Answer from the drawing. Dimensions are ordinates in mm from the lowest x, y and z of the part. Round coordinates to 2 decimals unless told otherwise and drop trailing zeros. Write each loop counter-clockwise with the first axis right and the second up, starting at its lowest first coordinate (ties: lowest second). Pieces come first, ordered by that corner, then holes. Notation, with made-up numbers: (10.25, 27.5) -> (48.25, 27.5) arc R9 ccw to (48.25, 38.5) -> close; hole circle Ø3 at (88.5, -13.5). An arc over 180 degrees is marked (long way). Return JSON: item names as keys, results as strings. Group by question number.
(1) A cutting plane is placed at C-C on z = 10.25. Give the vertices of the cut face in (x, y), then the cut area to 3 significant figures.
(2) Given pin 1 (6 mm diameter, centred on y = 1.5, z = 7, fed in from +X); pin 2 (1.5 mm diameter, centred on x = 4.5, z = 16.5, fed in from -Y); pin 3 (3 mm diameter, centred on x = 3, y = 13.5, fed in from +Z) (1 decimal), each flat-ended and moving along its own axis, determine where each tip first touches the part or whether it passes through.
(3) A cutting plane is placed at D-D on z = 21.75. Give the vertices of the cut face in (x, y).
(4) Straight lines are drawn through the part: line 1 (X direction, y = 7.62, z = 1.2); line 2 (Y direction, x = 14, z = 15) (1 decimal). For each, find the intervals that lie inside material, in ascending order.
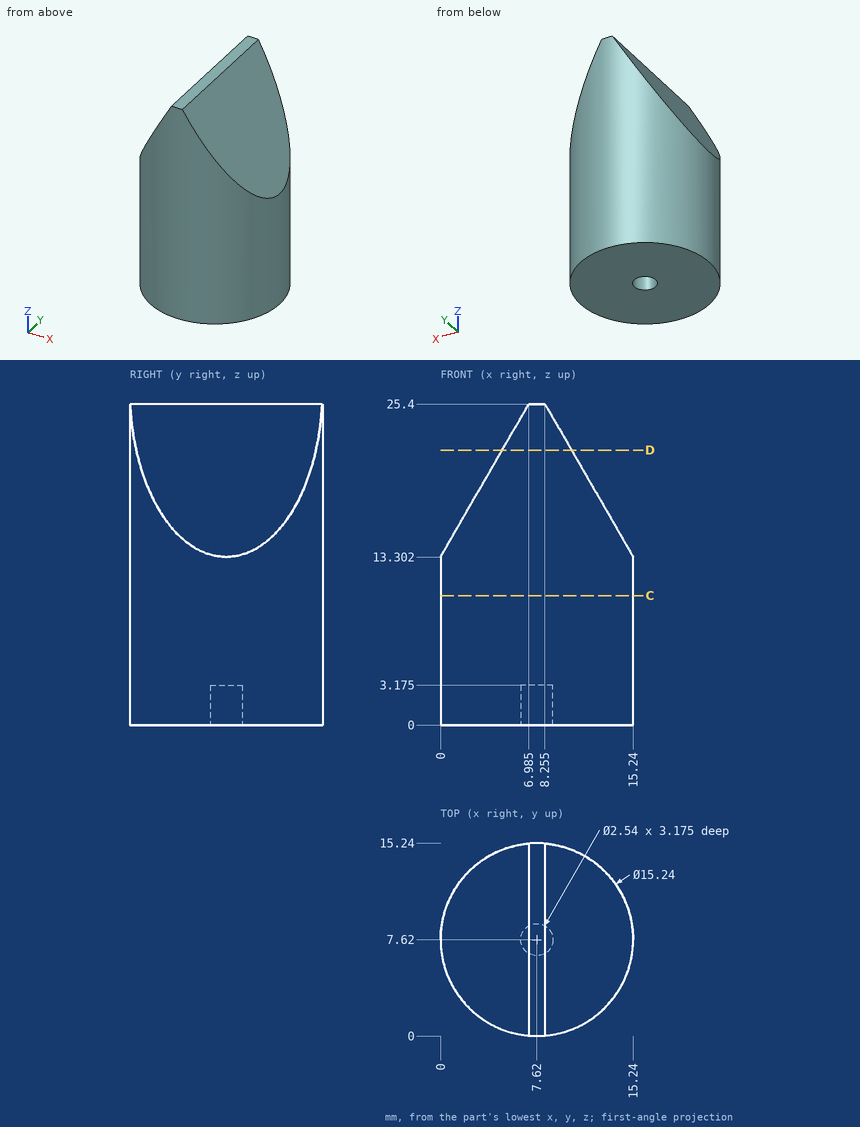
Checks:
{
 "1": {"outline": "circle Ø15.24 at (7.62, 7.62)", "area": "182 mm^2"},
 "2": {"pin 1": "stops at x = 14.57", "pin 2": "stops at y = 0.38", "pin 3": "stops at z = 21.1"},
 "3": {"outline": "(4.88, 0.51) arc R7.62 ccw to (10.36, 0.51) -> (10.36, 14.73) arc R7.62 ccw to (4.88, 14.73) -> close"},
 "4": {"line 1": "x = 0 to 6.35, 8.89 to 15.24", "line 2": "y = 3.5 to 11.8"}
}
